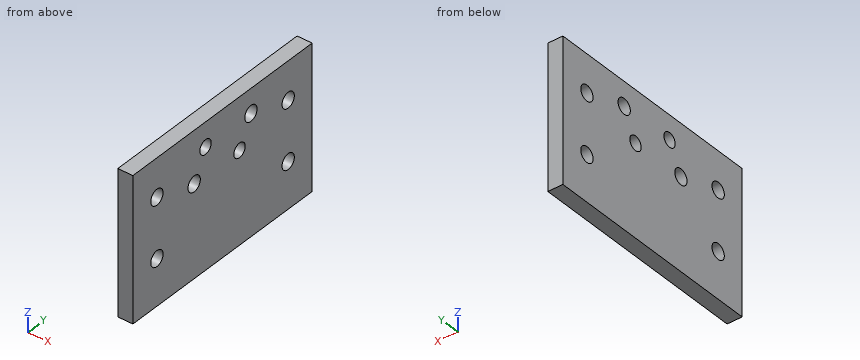
```python
from build123d import *

# Parameters (mm, degrees)
SKETCH1_R           = 3
SKETCH1_R_2         = 3.25755
BOSS_EXTRUDE1_DEPTH = 6.35
SKETCH2_W           = 94.8
SKETCH2_H           = 25.4
CUT_EXTRUDE1_DEPTH  = 6.35


with BuildPart() as part:
    # Sketch1 → Boss-Extrude1 (new body)
    with BuildSketch(Plane.YZ):
        Polygon((-47.4, -25), (-47.4, -69.8), (47.4, -69.8), (47.4, 16), (-47.4, 16), align=None)
        with Locations((-9, 5.8)):
            Circle(SKETCH1_R, mode=Mode.SUBTRACT)
        with Locations((-15, -5.8)):
            Circle(SKETCH1_R_2, mode=Mode.SUBTRACT)
        with Locations((9, -5.8)):
            Circle(SKETCH1_R, mode=Mode.SUBTRACT)
        with Locations((15, 5.8)):
            Circle(SKETCH1_R_2, mode=Mode.SUBTRACT)
        with Locations((-34.7, -57.1)):
            Circle(SKETCH1_R_2, mode=Mode.SUBTRACT)
        with Locations((34.7, -57.1)):
            Circle(SKETCH1_R_2, mode=Mode.SUBTRACT)
        with Locations((-34.7, -25)):
            Circle(SKETCH1_R_2, mode=Mode.SUBTRACT)
        with Locations((-34.7, 0)):
            Circle(SKETCH1_R_2, mode=Mode.SUBTRACT)
        with Locations((34.7, 0)):
            Circle(SKETCH1_R_2, mode=Mode.SUBTRACT)
        with Locations((34.7, -25)):
            Circle(SKETCH1_R_2, mode=Mode.SUBTRACT)
    extrude(amount=BOSS_EXTRUDE1_DEPTH)

    # Sketch2 → Cut-Extrude1 (cut)
    with BuildSketch(Plane.YZ.offset(6.35)):
        with Locations((0, -57.1)):
            Rectangle(SKETCH2_W, SKETCH2_H)
    extrude(amount=-CUT_EXTRUDE1_DEPTH, mode=Mode.SUBTRACT)


solid = part.part
```
Can you work these out from the model? Positions are in its coordinate system, mm. Coordinates: 2 decimals unless noted, no trailing zeros. Write each loop counter-clockwise with the first axis right and the second up, starting at its lowest first coordinate (ties: lowest second). Pieces come first, ordered by that corner, then holes. Notation, with made-up numbers: (52, 54) - (103, 54) arc R27 cw to (103, 89) - close; hole circle Ø8 at (47.5, 34.5). An arc over 180 degrees is marked (long way). Return JSON: item names as keys, results as strings.
Q1. If we section it at D-D (y = 36): Please give me the cut outline in (x, z).
Computed values:
{"outline": "(0, -44.4) - (6.35, -44.4) - (6.35, -27.99) - (0, -27.99) - close; (0, -22.01) - (6.35, -22.01) - (6.35, -2.99) - (0, -2.99) - close; (0, 2.99) - (6.35, 2.99) - (6.35, 16) - (0, 16) - close"}
Q2. Please list where these lines run through material, in increasing order: L1, parallel to Y at x = 5.75, z = 5.5; L2, parallel to Z at x = 3.5, y = 34.7; L3, parallel to Y at x = 2.5, z = -4.5. Write a range as from..to.
Computed values:
{"L1": "y = -47.4..-11.98, -6.02..11.76, 18.24..47.4", "L2": "z = -44.4..-28.26, -21.74..-3.26, 3.26..16", "L3": "y = -47.4..-17.99, -12.01..6.3, 11.7..47.4"}
Q3. If we section it at A-A (z = -5.8): Please give me the cut outline in (x, y).
Computed values:
{"outline": "(0, -47.4) - (6.35, -47.4) - (6.35, -18.26) - (0, -18.26) - close; (0, -11.74) - (6.35, -11.74) - (6.35, 6) - (0, 6) - close; (0, 12) - (6.35, 12) - (6.35, 47.4) - (0, 47.4) - close"}
Q4. If we section it at C-C (x = 1.25): Count the separate pieces of the cut face and the enclosed holes in it, then the cut area to 3 significant figures.
Computed values:
{"separate pieces": "1", "enclosed holes": "8", "area": "5,470 mm2"}
Q5. If we section it at B-B (y = -9): Please give me the cut outline in (x, z), then the cut area to 3 significant figures.
Computed values:
{"outline": "(0, -44.4) - (6.35, -44.4) - (6.35, 2.8) - (0, 2.8) - close; (0, 8.8) - (6.35, 8.8) - (6.35, 16) - (0, 16) - close", "area": "345 mm2"}
Q6. I'm going to push a flat-ended pin straight in: pin 1 Ø5 at (y, z) = (34.7, -25) entering from +X. Where does the tip first touch, or does it pass through?
Computed values:
{"pin 1": "passes through"}
